Read the model definition and answer for the solid it produces. Units are mm, in the model's axes. A direction names the side the tool comes from. Give positions to 0.01 mm unless a question says otherwise; leave off trailing zeros. Loops run counter-clockwise (first coordinate to the right, second up) from the corner with the lowest first, then second, coordinate; pieces in that order, holes last.
(1) Find section C-C, the plane z = 7.5. Write down the section's boundary in (x, y), then the cut area to 3 significant figures.
(2) Find section A-A, the plane y = 160.5. Write down the section's boundary in (x, z), then the cut area to 3 significant figures.
(3) Straight lines are drawn through the part: probe 1 along X at (y, z) = (240, 1.5); probe 2 along Z at (x, y) = (1.5, -35); probe 3 along Z at (x, y) = (-10.25, 133). For each, find the intervals that lie inside material, in ascending order.
(4) Determine the mould class of faces 1 (the face through (-12, -5, 0)), 2 (the face through (0, -5, -25)), 3 (the face through (15, -5, 0)) for opening direction Z: pulls with the +Z half, pulls with the -Z half, needs draft (parallel to the pull), parting line crosses it, or undercut.
(5) This flat-tipped pin is pushed along its axis until it touches: P1, Ø12, axis at x = -2.5, z = -19.5, coming from the +Y side. Where does it stop, or does it pass through?
(6) Which of the six approach directions +Z, -Z, +X, -X, +Y, -Y give full straight-line access (tool end or side, diameter ignored) to faces 4 (the face through (12, -5, 0)), 5 (the face through (0, -5, 25))?
(7) Find section B-B, the plane x = 2.5. Write down the section's boundary in (y, z), then the cut area to 3 significant figures.
```python
from build123d import *

# Parameters (mm, degrees)
F1_DEPTH = 366.5
F3_DEPTH = 50


with BuildPart() as f1:
    # F0 (on Front) → F1 (new body, symmetric)
    with BuildSketch(Plane.XZ):
        with BuildLine():
            ThreePointArc((15, 19), (13.2426406871, 23.2426406871), (9, 25))
            Line((9, 25), (-9, 25))
            ThreePointArc((-9, 25), (-13.2426406871, 23.2426406871), (-15, 19))
            Line((-15, 19), (-15, -19))
            ThreePointArc((-15, -19), (-13.2426406871, -23.2426406871), (-9, -25))
            Line((-9, -25), (9, -25))
            ThreePointArc((9, -25), (13.2426406871, -23.2426406871), (15, -19))
            Line((15, -19), (15, 19))
        make_face()
        with BuildLine():
            Line((-9, 22), (9, 22))
            ThreePointArc((9, 22), (11.1213203436, 21.1213203436), (12, 19))
            Line((12, 19), (12, -19))
            ThreePointArc((12, -19), (11.1213203436, -21.1213203436), (9, -22))
            Line((9, -22), (-9, -22))
            ThreePointArc((-9, -22), (-11.1213203436, -21.1213203436), (-12, -19))
            Line((-12, -19), (-12, 19))
            ThreePointArc((-12, 19), (-11.1213203436, 21.1213203436), (-9, 22))
        make_face(mode=Mode.SUBTRACT)
    extrude(amount=F1_DEPTH, both=True)

    # F2 (on face) → F3 (cut, through all)
    with BuildSketch(Plane.XY.offset(25)):
        Polygon((-9, -366.5), (-9, -360.5), (-15, -366.5), align=None)
        Polygon((9, -366.5), (9, -342.5), (-9, -360.5), (-9, -366.5), align=None)
        Polygon((15, -336.5), (9, -342.5), (9, -366.5), (15, -366.5), align=None)
        Polygon((-15, 366.5), (-9, 360.5), (-9, 366.5), align=None)
        Polygon((-9, 360.5), (9, 342.5), (9, 366.5), (-9, 366.5), align=None)
        Polygon((9, 342.5), (15, 336.5), (15, 366.5), (9, 366.5), align=None)
    extrude(amount=-F3_DEPTH, mode=Mode.SUBTRACT)


solid = f1.part
```
Entries:
1. outline: (-15, -366.5) - (-12, -363.5) - (-12, 363.5) - (-15, 366.5) - close; (12, -339.5) - (15, -336.5) - (15, 336.5) - (12, 339.5) - close
1. area: 4,220 mm2
2. outline: (-15, -19) arc R6 ccw to (-9, -25) - (9, -25) arc R6 ccw to (15, -19) - (15, 19) arc R6 ccw to (9, 25) - (-9, 25) arc R6 ccw to (-15, 19) - close; hole (-12, -19) arc R3 ccw to (-9, -22) - (9, -22) arc R3 ccw to (12, -19) - (12, 19) arc R3 ccw to (9, 22) - (-9, 22) arc R3 ccw to (-12, 19) - close
2. area: 421 mm2
3. probe 1: x = -15 to -12, 12 to 15
3. probe 2: z = -25 to -22, 22 to 25
3. probe 3: z = -24.87 to -21.73, 21.73 to 24.87
4. face 1: undercut
4. face 2: pulls with the -Z half
4. face 3: needs draft
5. P1: stops at y = 359.45
6. face 4: +Y, -Y
6. face 5: +Z, +X, -X, +Y, -Y
7. outline: (-349, -25) - (349, -25) - (349, -22) - (-349, -22) - close; (-349, 22) - (349, 22) - (349, 25) - (-349, 25) - close
7. area: 4,190 mm2
